Source: three-view drawing plus pictorial views. Frame: mm from the lowest corner of the part. Round coordinates to 2 decimals unless told otherwise and drop trailing zeros. Loops run counter-clockwise (first coordinate to the right, second up) from the corner with the lowest first, then second, coordinate; pieces in that order, holes last. Notation, with made-up numbers: (48.25, 16.5) -> (62.25, 16.5) arc R32 cw to (62.25, 47.5) -> close; hole circle Ø7 at (51, 65). An arc over 180 degrees is marked (long way). Answer in a Markdown table with one row per item. Add a question column.
Q1. Section B-B, the plane y = 1. Output: boundary loops of the cut face in (x, z).
Q2. Section A-A, the plane z = 2.5. Give the number of separate pieces and of enclosed holes in the cut face, and give its area (4 significant figures).
Q3. Ray query, L1, parallel to X at y = 8, z = 2.5; L2, parallel to X at y = 11.25, z = 8.5 (1 decimal); L3, parallel to Y at x = 60, z = 2. Return the intervals inside material, ascending. Write a range as from..to.
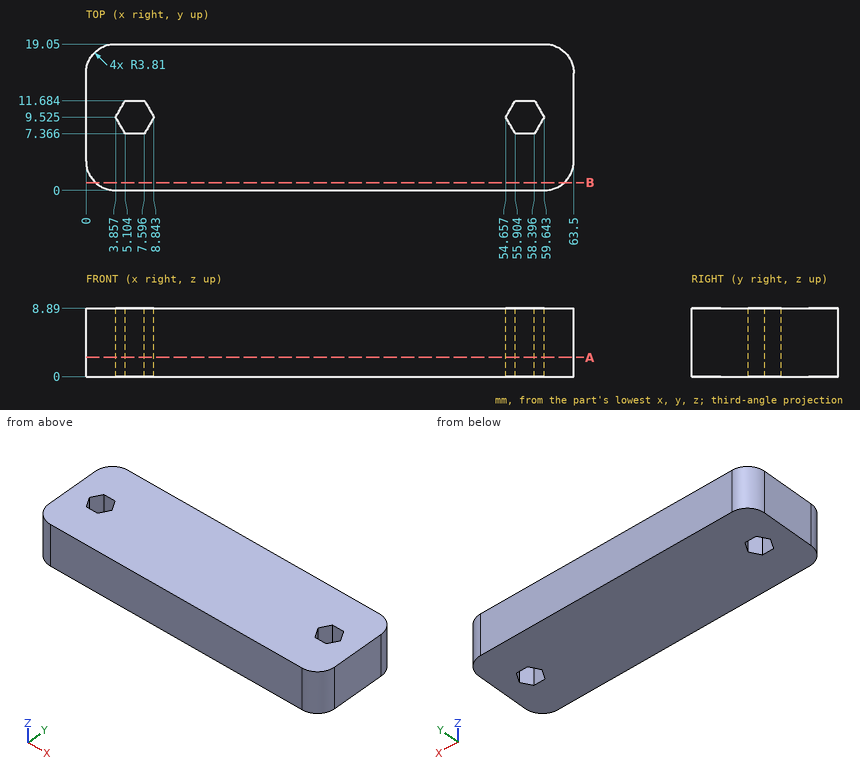
Answer block:
| question | item | result |
|---|---|---|
| 1 | outline | (1.24, 0) -> (62.26, 0) -> (62.26, 8.89) -> (1.24, 8.89) -> close |
| 2 | separate pieces | 1 |
| 2 | enclosed holes | 2 |
| 2 | area | 1,165 mm^2 |
| 3 | L1 | 0..4.74, 7.96..55.54, 58.76..63.5 |
| 3 | L2 | 0..4.9, 7.8..55.7, 58.6..63.5 |
| 3 | L3 | 0.01..19.04 |
